```python
from build123d import *
from build123d import SkipClean  # not in build123d's __all__


with BuildPart() as f1:
    # F0 (on Front) → F1 (revolve)
    with BuildSketch(Plane.XZ):
        with BuildLine():
            Line((-3.5, 324), (-3.5, 1))
            Line((-3.5, 1), (-2.5, 0))
            Line((-2.5, 0), (0, 0))
            Line((0, 0), (0, 317.4226497308))
            Line((0, 317.4226497308), (-1, 318))
            Line((-1, 318), (-1, 323.5))
            ThreePointArc((-1, 323.5), (-1.4393398282, 324.5606601718), (-2.5, 325))
            ThreePointArc((-2.5, 325), (-3.2071067812, 324.7071067812), (-3.5, 324))
        make_face()
    revolve(axis=Axis((0, 0, 158.7113248654), (0, 0, -1)))

    # F2 (on Front) → F3 (revolve, cut)
    with BuildSketch(Plane.XZ):
        Polygon((-1, 319), (-2.1547005384, 317), (10.5847728806, 317), (10.5847728806, 319), align=None)
    revolve(axis=Axis((7.4317818913, 0, 317), (1, 0, 0)), mode=Mode.SUBTRACT)

    # F4 (on Front) → F5 (revolve, cut)
    with BuildSketch(Plane.XZ):
        Polygon((7.5055534995, 311.4226497308), (1.3094010768, 315), (-1, 315), (-1, 316.3333333333), (-2.1547005384, 317), (-2.1547005384, 314.6905989232), (6.5055534995, 309.6905989232), align=None)
        Polygon((-1, 315), (1.3094010768, 315), (-1, 316.3333333333), align=None)
    with SkipClean():  # cleaning this boolean's faces spoils the solid; the shape is the same uncleaned
        revolve(axis=Axis((2.6754264805, 0, 314.2113248654), (0.8660254038, 0, -0.5)), mode=Mode.SUBTRACT)


solid = f1.part
```
The model under review builds one solid part; all positions refer to its coordinate system, in mm. Round coordinates to 2 decimals unless told otherwise and drop trailing zeros. Order: outer loops, then holes, each group sorted by start corner. A loop starts at its lowest first (then second) coordinate and runs counter-clockwise, first axis right, second up. Notation, with made-up numbers: (88, 13) - (116, 13) arc R28 ccw to (116, 42) - close; hole circle Ø3 at (45, 58.25). An arc over 180 degrees is marked (long way). Answer in a Markdown table with one row per item.
(1) Take a section at A-A on z = 174. Write out the cut boundary in (x, y).
Result set:
| item | result |
|---|---|
| outline | circle Ø7 at (0, 0) |
(2) Clearance check with flat-ended pins moving along their axes: P1, Ø1.2, axis at x = 0, y = 0, coming from the +Z side; P2, Ø2, axis at y = -2, z = 72, coming from the +X side. State where each tip first meets the part, or that it passes through.
Result set:
| item | result |
|---|---|
| P1 | stops at z = 313.79 |
| P2 | stops at x = 3.35 |
(3) For line 1 (X direction, y = 0, z = 321.1); line 2 (Y direction, x = 0.5, z = 283), list the stretches that pass through material, from the lowest coordinate up. Write a range as from..to.
Result set:
| item | result |
|---|---|
| line 1 | x = -3.5..-1, 1..3.5 |
| line 2 | y = -3.46..3.46 |
